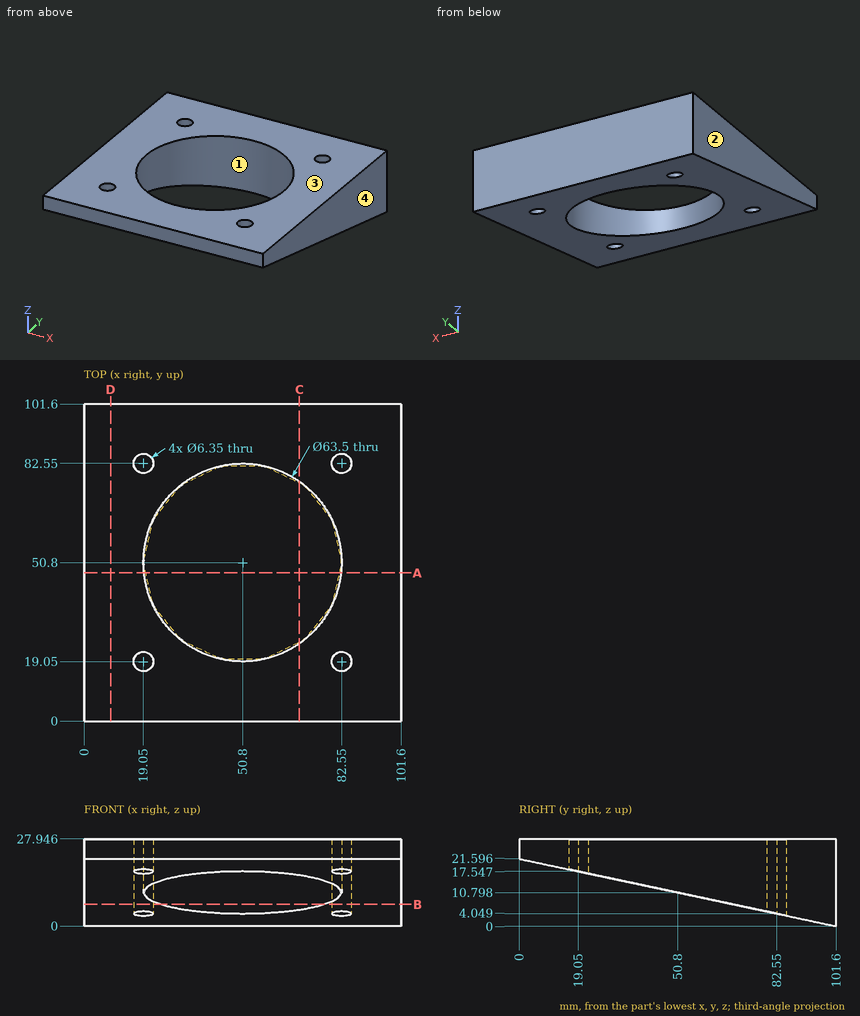
Geometry check sheet. Reference: drawing and pictorial views, mm from the part's lowest x, y, z. Coordinates: 2 decimals unless noted, no trailing zeros. Order: outer loops, then holes, each group sorted by start corner. A loop starts at its lowest first (then second) coordinate and runs counter-clockwise, first axis right, second up.
1. Scan lines: line 1 (Y direction, x = 53, z = 25.75); line 2 (X direction, y = 37, z = 14.75) (1 decimal); line 3 (X direction, y = 39.5, z = 13.25). Record each from-to range of solid material in increasing order.
Results found:
line 1: y = 0 to 19.13, 82.47 to 101.6
line 2: x = 0 to 22.2, 79.4 to 101.6
line 3: x = 0 to 21.13, 80.47 to 101.6
2. Sectioned sample at C-C, the plane x = 69. Record the cut outline in (y, z) (1 decimal), and give its area (3 significant figures).
Results found:
outline: (0, 21.6) - (24.8, 16.3) - (24.8, 27.9) - (0, 27.9) - close; (76.8, 5.3) - (101.6, 0) - (101.6, 27.9) - (76.8, 27.9) - close
area: 850 mm2
3. Sectioned sample at B-B, the plane z = 7. Give the number of separate pieces and of enclosed holes in the cut face, and give its area (3 significant figures).
Results found:
separate pieces: 1
enclosed holes: 2
area: 2,770 mm2
4. Release check for a two-part mould opening along X. For the marked faces 1, 2, 3 and 4 record: +X half, -X half, draft (parallel to the pull), parting line (faces both ways), or undercut.
Results found:
face 1: undercut
face 2: -X half
face 3: draft
face 4: +X half
5. Sectioned sample at A-A, the plane y = 47.5. Record the cut outline in (x, z) (1 decimal).
Results found:
outline: (0, 11.5) - (19.2, 11.5) - (19.2, 27.9) - (0, 27.9) - close; (82.4, 11.5) - (101.6, 11.5) - (101.6, 27.9) - (82.4, 27.9) - close
6. Sectioned sample at D-D, the plane x = 8.5. Record the cut outline in (y, z) (1 decimal), and give its area (3 significant figures).
Results found:
outline: (0, 21.6) - (101.6, 0) - (101.6, 27.9) - (0, 27.9) - close
area: 1,740 mm2
